```python
from build123d import *

# Parameters (mm, degrees)
SKETCH1_W           = 63.5
SKETCH1_H           = 35
BOSS_EXTRUDE1_DEPTH = 12
SKETCH3_W           = 26.4
SKETCH3_H           = 35
CUT_EXTRUDE2_DEPTH  = 5
SKETCH4_W           = 2.6
SKETCH4_H           = 35
CUT_EXTRUDE3_DEPTH  = 1.3
SKETCH5_W           = 18.55
SKETCH5_H           = 35
CUT_EXTRUDE4_DEPTH  = 13
SKETCH6_W           = 18.55
SKETCH6_H           = 35
CUT_EXTRUDE5_DEPTH  = 13
SKETCH7_R           = 2.5
CUT_EXTRUDE6_DEPTH  = 36
SKETCH8_R           = 2.5
CUT_EXTRUDE7_DEPTH  = 36
SKETCH12_W          = 26.4
SKETCH12_H          = 10
BOSS_EXTRUDE2_DEPTH = 27
SKETCH13_W          = 20
SKETCH13_H          = 19.5
CUT_EXTRUDE8_DEPTH  = 11
SKETCH14_W          = 27
SKETCH14_H          = 3
CUT_EXTRUDE9_DEPTH  = 27.4
SKETCH18_W          = 2.6
SKETCH18_H          = 1.3
CUT_EXTRUDE12_DEPTH = 28
SKETCH19_W          = 10
SKETCH19_H          = 5
CUT_EXTRUDE13_DEPTH = 27.4
SKETCH20_W          = 2.5
SKETCH20_H          = 5
CUT_EXTRUDE14_DEPTH = 27.4
CUT_EXTRUDE15_DEPTH = 27.4
SKETCH24_W          = 26.4
SKETCH24_H          = 2
CUT_EXTRUDE18_DEPTH = 5
SKETCH25_W          = 26.4
SKETCH25_H          = 7
CUT_EXTRUDE19_DEPTH = 8
SKETCH26_R          = 1.3
CUT_EXTRUDE20_DEPTH = 56


with BuildPart() as part:
    # Sketch1 → Boss-Extrude1 (new body)
    with BuildSketch(Plane(origin=(0, 0, 0), x_dir=(1, 0, 0), z_dir=(0, 1, 0))):
        with Locations((0, 17.5)):
            Rectangle(SKETCH1_W, SKETCH1_H)
    extrude(amount=BOSS_EXTRUDE1_DEPTH)

    # Sketch3 → Cut-Extrude2 (cut)
    with BuildSketch(Plane.XZ):
        with Locations((0, -17.5)):
            Rectangle(SKETCH3_W, SKETCH3_H)
    extrude(amount=-CUT_EXTRUDE2_DEPTH, mode=Mode.SUBTRACT)

    # Sketch4 → Cut-Extrude3 (cut)
    with BuildSketch(Plane.XZ.offset(-5)):
        with Locations((-4.5, -17.5)):
            Rectangle(SKETCH4_W, SKETCH4_H)
        with Locations((4.5, -17.5)):
            Rectangle(SKETCH4_W, SKETCH4_H)
    extrude(amount=-CUT_EXTRUDE3_DEPTH, mode=Mode.SUBTRACT)

    # Sketch5 → Cut-Extrude4 (cut, through all)
    with BuildSketch(Plane.XZ):
        with Locations((-22.475, -17.5)):
            Rectangle(SKETCH5_W, SKETCH5_H)
    extrude(amount=-CUT_EXTRUDE4_DEPTH, mode=Mode.SUBTRACT)

    # Sketch6 → Cut-Extrude5 (cut, through all)
    with BuildSketch(Plane.XZ):
        with Locations((22.475, -17.5)):
            Rectangle(SKETCH6_W, SKETCH6_H)
    extrude(amount=-CUT_EXTRUDE5_DEPTH, mode=Mode.SUBTRACT)

    # Sketch7 → Cut-Extrude6 (cut, through all)
    with BuildSketch(Plane.XY):
        with Locations((-9, 8.5)):
            Circle(SKETCH7_R)
    extrude(amount=-CUT_EXTRUDE6_DEPTH, mode=Mode.SUBTRACT)

    # Sketch8 → Cut-Extrude7 (cut, through all)
    with BuildSketch(Plane.XY):
        with Locations((9, 8.5)):
            Circle(SKETCH8_R)
    extrude(amount=-CUT_EXTRUDE7_DEPTH, mode=Mode.SUBTRACT)

    # Sketch12 → Boss-Extrude2 (add)
    with BuildSketch(Plane.XY):
        with Locations((0, 10)):
            Rectangle(SKETCH12_W, SKETCH12_H)
    extrude(amount=BOSS_EXTRUDE2_DEPTH)

    # Sketch13 → Cut-Extrude8 (cut, through all)
    with BuildSketch(Plane(origin=(0, 15, 0), x_dir=(1, 0, 0), z_dir=(0, 1, 0))):
        with Locations((0, -14.75)):
            Rectangle(SKETCH13_W, SKETCH13_H)
    extrude(amount=-CUT_EXTRUDE8_DEPTH, mode=Mode.SUBTRACT)

    # Sketch14 → Cut-Extrude9 (cut, through all)
    with BuildSketch(Plane.ZY.offset(13.2)):
        with Locations((13.5, 13.5)):
            Rectangle(SKETCH14_W, SKETCH14_H)
    extrude(amount=-CUT_EXTRUDE9_DEPTH, mode=Mode.SUBTRACT)

    # Sketch18 → Cut-Extrude12 (cut, through all)
    with BuildSketch(Plane(origin=(0, 0, 0), x_dir=(-1, 0, 0), z_dir=(0, 0, -1))):
        with Locations((4.5, 5.65)):
            Rectangle(SKETCH18_W, SKETCH18_H)
        with Locations((-4.5, 5.65)):
            Rectangle(SKETCH18_W, SKETCH18_H)
    extrude(amount=-CUT_EXTRUDE12_DEPTH, mode=Mode.SUBTRACT)

    # Sketch19 → Cut-Extrude13 (cut, through all)
    with BuildSketch(Plane.ZY.offset(13.2)):
        with Locations((9, 7.5)):
            Rectangle(SKETCH19_W, SKETCH19_H)
    extrude(amount=-CUT_EXTRUDE13_DEPTH, mode=Mode.SUBTRACT)

    # Sketch20 → Cut-Extrude14 (cut, through all)
    with BuildSketch(Plane.ZY.offset(13.2)):
        with Locations((25.75, 7.5)):
            Rectangle(SKETCH20_W, SKETCH20_H)
    extrude(amount=-CUT_EXTRUDE14_DEPTH, mode=Mode.SUBTRACT)

    # Sketch21 → Cut-Extrude15 (cut, through all)
    with BuildSketch(Plane.ZY.offset(13.2)):
        Polygon((14, 10), (14.647047613, 7.585185434), (23.6593, 10), (24.5, 10), (24.5, 5), (14, 5), align=None)
    extrude(amount=-CUT_EXTRUDE15_DEPTH, mode=Mode.SUBTRACT)

    # Sketch24 → Cut-Extrude18 (cut)
    with BuildSketch(Plane.XZ.offset(-5)):
        with Locations((0, 3)):
            Rectangle(SKETCH24_W, SKETCH24_H)
    extrude(amount=-CUT_EXTRUDE18_DEPTH, mode=Mode.SUBTRACT)

    # Sketch25 → Cut-Extrude19 (cut, through all)
    with BuildSketch(Plane(origin=(0, 12, 0), x_dir=(1, 0, 0), z_dir=(0, 1, 0))):
        with Locations((0, 31.5)):
            Rectangle(SKETCH25_W, SKETCH25_H)
    extrude(amount=-CUT_EXTRUDE19_DEPTH, mode=Mode.SUBTRACT)

    # Sketch26 → Cut-Extrude20 (cut, through all)
    with BuildSketch(Plane(origin=(0, 0, -28), x_dir=(-1, 0, 0), z_dir=(0, 0, -1))):
        with Locations((4.5, 6.3)):
            Circle(SKETCH26_R)
        with Locations((-4.5, 6.3)):
            Circle(SKETCH26_R)
    extrude(amount=-CUT_EXTRUDE20_DEPTH, mode=Mode.SUBTRACT)


solid = part.part
```
Geometry: final body of the model. Coordinates: model frame, mm. A direction names the side the tool comes from. Coordinates: 2 decimals unless noted, no trailing zeros. Order: outer loops, then holes, each group sorted by start corner. A loop starts at its lowest first (then second) coordinate and runs counter-clockwise, first axis right, second up. Notation, with made-up numbers: (42, -37.5) - (48, -37.5) arc R9 cw to (48, -29.5) - close; hole circle Ø10 at (25.5, -21.75). An arc over 180 degrees is marked (long way). Write each question's results on one line, items separated by ' | '.
(1) Section query A-A, the plane x = 0. Return the cut outline in (y, z).
Values found:
outline: (5, -28) - (12, -28) - (12, 5) - (10, 5) - (10, 2) - (5, 2) - close; (10, 24.5) - (12, 24.5) - (12, 27) - (10, 27) - close
(2) Line query: line 1 (Y direction, x = 9, z = -13.25); line 2 (X direction, y = 11.75, z = 23); line 3 (X direction, y = 7.75, z = -10.5). Output: solid intervals per line, ascending. Write a range as [from, to].
Values found:
line 1: y = [5, 6], [11, 12] | line 2: x = [-13.2, -10], [10, 13.2] | line 3: x = [-13.2, -11.38], [-6.62, 6.62], [11.38, 13.2]
(3) Set-up query: faces 3 (the face through (0, 10, 26)), 4 (the face through (-9, 9, 0)), 5 (the face through (-3.2, 6, -13)), 6 (the face through (-10, 10, 15)), 7 (the face through (11.58, 8.81, 14.32)). Return all of +Z, -Z, +X, -X, +Y, -Y with unobstructed straight access to the full face (end or side cutting, diameter ignored); none if empty.
Values found:
face 3: +Z, +X, -X, -Y | face 4: -Z | face 5: +Z, -Z, -Y | face 6: +Y, -Y | face 7: +X, -X, -Y
(4) Section query C-C, the plane z = 0.5. Return the cut outline in (x, y), plus the area to 3 significant figures.
Values found:
outline: (-13.2, 5) - (-5.8, 5) - (-5.8, 6.3) arc R1.3 cw to (-3.2, 6.3) - (-3.2, 5) - (3.2, 5) - (3.2, 6.3) arc R1.3 cw to (5.8, 6.3) - (5.8, 5) - (13.2, 5) - (13.2, 12) - (-13.2, 12) - close | area: 173 mm²
(5) Section query D-D, the plane x = -10.5. Return the cut outline in (y, z), plus the area to 3 significant figures.
Values found:
outline: (5, -28) - (6.5, -28) - (6.5, 0) - (10.5, 0) - (10.5, -28) - (12, -28) - (12, 27) - (10, 27) - (10, 23.66) - (7.59, 14.65) - (10, 14) - (10, 2) - (5, 2) - close | area: 160 mm²
(6) Section query B-B, the plane z = -11. Return the cut outline in (x, y).
Values found:
outline: (-13.2, 5) - (-5.8, 5) - (-5.8, 6.3) arc R1.3 cw to (-3.2, 6.3) - (-3.2, 5) - (3.2, 5) - (3.2, 6.3) arc R1.3 cw to (5.8, 6.3) - (5.8, 5) - (13.2, 5) - (13.2, 12) - (-13.2, 12) - close; hole circle Ø5 at (-9, 8.5); hole circle Ø5 at (9, 8.5)
(7) First-contact query: pin 1 Ø1 at (x, y) = (-9, 9) entering from -Z; pin 2 Ø13 at (x, z) = (4.5, 10) entering from -Y; pin 3 Ø3.5 at (y, z) = (9.5, 12.5) entering from -X; pin 4 Ø2.5 at (x, y) = (-6, 8) entering from +Z. Flat tips, straight axial feed; report the tip coordinate or a pass-through.
Values found:
pin 1: stops at z = 0 | pin 2: stops at y = 10 | pin 3: stops at x = -13.2 | pin 4: stops at z = 2
(8) Mould query, pull axis X, two halves, no side actions, for faces 1 (the face through (0, 5, -13)), 2 (the face through (0, 11, 5)). Classes: +X half, -X half, draft (parallel to the pull), parting line (faces both ways), or undercut.
Values found:
face 1: draft | face 2: undercut
